from build123d import *

# Parameters (mm, degrees)
SKETCH_W        = 40
SKETCH_H        = 45
PAD_DEPTH       = 10
SKETCH001_R     = 1.971831
SKETCH001_R_2   = 2.210302
POCKET_DEPTH    = 10
SKETCH002_W     = 40
SKETCH002_H     = 33
POCKET001_DEPTH = 6
SKETCH003_R     = 1.6
POCKET002_DEPTH = 5
SKETCH004_W     = 5
SKETCH004_H     = 12.28172
POCKET003_DEPTH = 3.6
FILLET_R        = 6


with BuildPart() as part:
    # Sketch → Pad (new body)
    with BuildSketch(Plane.XY):
        with Locations((20, 22.5)):
            Rectangle(SKETCH_W, SKETCH_H)
    extrude(amount=PAD_DEPTH)

    # Sketch001 (on Face6 of Pad) → Pocket (cut)
    with BuildSketch(Plane.XY.offset(10)):
        with Locations((10, 7.5)):
            Circle(SKETCH001_R)
        with Locations((30, 7.5)):
            Circle(SKETCH001_R_2)
    extrude(amount=-POCKET_DEPTH, mode=Mode.SUBTRACT)

    # Sketch002 (on Face5 of Pocket) → Pocket001 (cut)
    with BuildSketch(Plane.XY.offset(10)):
        with Locations((20, 28.5)):
            Rectangle(SKETCH002_W, SKETCH002_H)
    extrude(amount=-POCKET001_DEPTH, mode=Mode.SUBTRACT)

    # Sketch003 (on Face7 of Pocket001) → Pocket002 (cut)
    with BuildSketch(Plane.XY.offset(4)):
        with Locations((14, 21.999999)):
            Circle(SKETCH003_R)
        with Locations((26, 22)):
            Circle(SKETCH003_R)
    extrude(amount=-POCKET002_DEPTH, mode=Mode.SUBTRACT)

    # Sketch004 (on Face5 of Pocket002) → Pocket003 (cut)
    with BuildSketch(Plane.XY.offset(10)):
        with Locations((20, 6.14086)):
            Rectangle(SKETCH004_W, SKETCH004_H)
    extrude(amount=-POCKET003_DEPTH, mode=Mode.SUBTRACT)

    # Fillet
    fillet_edges = [part.edges().sort_by_distance(p)[0] for p in [
        (40, 0, 5),
        (0, 0, 5),
        (40, 45, 2),
        (0, 45, 2),
    ]]
    fillet(fillet_edges, radius=FILLET_R)


solid = part.part
For this review, take the finished solid that the model builds, in its own axes (mm). A direction names the side the tool comes from. Coordinates: 2 decimals unless noted, no trailing zeros. Write each loop counter-clockwise with the first axis right and the second up, starting at its lowest first coordinate (ties: lowest second). Pieces come first, ordered by that corner, then holes. Notation, with made-up numbers: (72.5, 71) -> (101.5, 71) arc R20 ccw to (101.5, 90) -> close; hole circle Ø2 at (14.25, 32.25). An arc over 180 degrees is marked (long way). Write each question's results on one line, items separated by ' | '. Start each with the question number.
1) For faces 4 (the face through (20, 6, 6.4)), 5 (the face through (20, 45, 2)), 6 (the face through (20, 29, 4)), list the 3-axis set-ups (+Z, -Z, +X, -X, +Y, -Y) from which the entire face can be reached by the end or side of a thin tool; tool diameter is ignored.
2) Consider section B-B (x = 30). Write out the cut boundary in (y, z), plus the area to 3 significant figures.
3) Consider section D-D (x = 10). Write out the cut boundary in (y, z), plus the area to 3 significant figures.
4) Insertion check: pin 1 (4 mm diameter, centred on x = 30, y = 7.5, fed in from +Z); pin 2 (2 mm diameter, centred on x = 25.5, y = 24, fed in from +Z); pin 3 (4 mm diameter, centred on x = 20, y = 4, fed in from +Z). Each pin has a flat end and moves straight along its axis. Give the tip position at first contact, or say it passes through.
5) Consider section C-C (z = 2.25). Write out the cut boundary in (x, y).
6) Consider section A-A (z = 9). Write out the cut boundary in (x, y), plus the area to 3 significant figures.
7) Wall thickness on L1, parallel to Y at x = 10, z = 7; L2, parallel to Y at x = 26, z = 1.4; L3, parallel to X at y = 8.5, z = 4.25: over which ranges is each line inside the solid? List them lowest first. Write a range as [from, to].
8) The part is to be moulded in two halves that separate along X. For faces 1 (the face through (1.711, 43.196, 2.028)), 2 (the face through (11.82, 6.74, 5.07)), 3 (the face through (9, 5, 10)), say which applies: +X half, -X half, draft (parallel to the pull), parting line (faces both ways), or undercut.
Geometry says:
1) face 4: +Z, +Y, -Y | face 5: +Z, -Z, +X, -X, +Y | face 6: +Z, +X, -X, +Y
2) outline: (0, 0) -> (5.29, 0) -> (5.29, 10) -> (0, 10) -> close; (9.71, 0) -> (45, 0) -> (45, 4) -> (12, 4) -> (12, 10) -> (9.71, 10) -> close | area: 208 mm^2
3) outline: (0, 0) -> (5.53, 0) -> (5.53, 10) -> (0, 10) -> close; (9.47, 0) -> (45, 0) -> (45, 4) -> (12, 4) -> (12, 10) -> (9.47, 10) -> close | area: 213 mm^2
4) pin 1: through | pin 2: z = 4 | pin 3: z = 6.4
5) outline: (0, 6) arc R6 ccw to (6, 0) -> (34, 0) arc R6 ccw to (40, 6) -> (40, 39) arc R6 ccw to (34, 45) -> (6, 45) arc R6 ccw to (0, 39) -> close; hole circle Ø3.94 at (10, 7.5); hole circle Ø3.2 at (14, 22); hole circle Ø3.2 at (26, 22); hole circle Ø4.42 at (30, 7.5)
6) outline: (0, 6) arc R6 ccw to (6, 0) -> (17.5, 0) -> (17.5, 12) -> (0, 12) -> close; (22.5, 0) -> (34, 0) arc R6 ccw to (40, 6) -> (40, 12) -> (22.5, 12) -> close; hole circle Ø3.94 at (10, 7.5); hole circle Ø4.42 at (30, 7.5) | area: 377 mm^2
7) L1: [0, 5.53], [9.47, 12] | L2: [0, 20.4], [23.6, 45] | L3: [0, 8.3], [11.7, 28.03], [31.97, 40]
8) face 1: -X half | face 2: undercut | face 3: draft
